Model file for the job. Use its own axes, mm. Face numbers are marked on the shaded views. Give positions to 0.01 mm unless a question says otherwise; leave off trailing zeros. Order: outer loops, then holes, each group sorted by start corner. A loop starts at its lowest first (then second) coordinate and runs counter-clockwise, first axis right, second up. Notation, with made-up numbers: (-23.75, 56) - (5.25, 56) arc R26 ccw to (5.25, 71) - close; hole circle Ø10 at (-34.75, 65.5). An arc over 180 degrees is marked (long way). Use CSV: the item, a comma, the result in double quotes. Start each with the question number.
(1) Band-saw the part on B-B, the plane x = -2. Give the cut face in (y, z), then the cut area to 3 significant figures.
(2) Probe L1, parallel to Z at x = 45.5, y = 23.25; L2, parallel to X at y = 23.5, z = 31; L3, parallel to Y at x = -7, z = -7.5. List the from-to ranges inside material, lowest first.
(3) Pull direction X, two halves, no side cores. Call the marked faces 1, 2, 3 and 4: +X half, -X half, draft (parallel to the pull), parting line (faces both ways), or undercut.
(4) Band-saw the part on C-C, the plane z = -17.5. Give the cut face in (x, y), then the cut area to 3 significant figures.
(5) Band-saw the part on A-A, the plane y = 21. Give the cut face in (x, z).
(6) Drop a flat-ended pin along its axis: pin 1 Ø10 at (x, z) = (-31.5, 21.5) entering from +Y. Give the stop position or say it passes through.
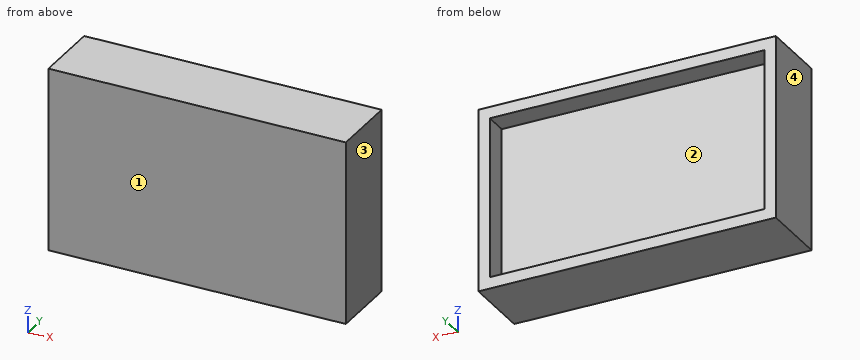
from build123d import *

# Parameters (mm, degrees)
SKETCH2_W           = 130
SKETCH2_H           = 80
BOSS_EXTRUDE1_DEPTH = 25
SKETCH5_W           = 120
SKETCH5_H           = 70
CUT_EXTRUDE1_DEPTH  = 10
SKETCH6_W           = 130
SKETCH6_H           = 80
BOSS_EXTRUDE2_DEPTH = 5


with BuildPart() as part:
    # Sketch2 → Boss-Extrude1 (new body)
    with BuildSketch(Plane(origin=(0, 0, 0), x_dir=(1, 0, 0), z_dir=(0, 1, 0))):
        Rectangle(SKETCH2_W, SKETCH2_H)
    extrude(amount=BOSS_EXTRUDE1_DEPTH)

    # Sketch5 → Cut-Extrude1 (cut)
    with BuildSketch(Plane(origin=(0, 25, 0), x_dir=(1, 0, 0), z_dir=(0, 1, 0))):
        Rectangle(SKETCH5_W, SKETCH5_H)
    extrude(amount=-CUT_EXTRUDE1_DEPTH, mode=Mode.SUBTRACT)

    # Sketch6 → Boss-Extrude2 (add)
    with BuildSketch(Plane(origin=(0, 0, 0), x_dir=(-1, 0, 0), z_dir=(0, -1, 0))):
        Rectangle(SKETCH6_W, SKETCH6_H)
    extrude(amount=BOSS_EXTRUDE2_DEPTH)


solid = part.part
Answer block:
1,outline,"(-5, -40) - (25, -40) - (25, -35) - (15, -35) - (15, 35) - (25, 35) - (25, 40) - (-5, 40) - close"
1,area,"1,700 mm2"
2,L1,"z = -40 to -35, 35 to 40"
2,L2,"x = -65 to -60, 60 to 65"
2,L3,"y = -5 to 15"
3,face 1,"draft"
3,face 2,"undercut"
3,face 3,"+X half"
3,face 4,"-X half"
4,outline,"(-65, -5) - (65, -5) - (65, 25) - (60, 25) - (60, 15) - (-60, 15) - (-60, 25) - (-65, 25) - close"
4,area,"2,700 mm2"
5,outline,"(-65, -40) - (65, -40) - (65, 40) - (-65, 40) - close; hole (-60, -35) - (60, -35) - (60, 35) - (-60, 35) - close"
6,pin 1,"stops at y = 15"
